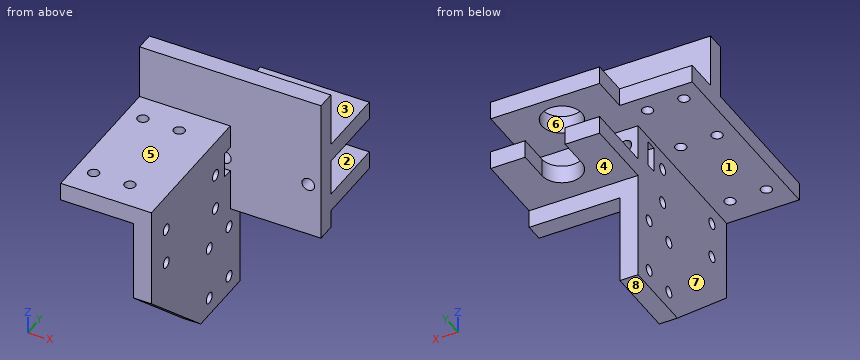
```python
from build123d import *

# Parameters (mm, degrees)
BOSS_EXTRUDE1_DEPTH = 10
SKETCH2_W           = 40
SKETCH2_H           = 10
BOSS_EXTRUDE2_DEPTH = 18.71
BOSS_EXTRUDE3_DEPTH = 80
SKETCH5_W           = 10
SKETCH5_H           = 90
BOSS_EXTRUDE4_DEPTH = 50
CUT_EXTRUDE1_DEPTH  = 10
SKETCH7_W           = 60
SKETCH7_H           = 10
BOSS_EXTRUDE5_DEPTH = 39
SKETCH8_R           = 3.5
CUT_EXTRUDE2_DEPTH  = 10
CUT_EXTRUDE3_DEPTH  = 10
SKETCH10_R          = 11
SKETCH10_R_2        = 3
CUT_EXTRUDE4_DEPTH  = 10
SKETCH11_R          = 3
CUT_EXTRUDE5_DEPTH  = 10
CUT_EXTRUDE6_START  = -10
CUT_EXTRUDE6_DEPTH  = 10


with BuildPart() as part:
    # Sketch1 → Boss-Extrude1 (new body)
    with BuildSketch(Plane(origin=(0, 0, 0), x_dir=(1, 0, 0), z_dir=(0, 1, 0))):
        Polygon((0, 0), (100, 0), (100, 80), (40, 80), (40, 40), (0, 40), align=None)
    extrude(amount=BOSS_EXTRUDE1_DEPTH)

    # Sketch2 → Boss-Extrude2 (add)
    with BuildSketch(Plane(origin=(0, 10, 0), x_dir=(1, 0, 0), z_dir=(0, 1, 0))):
        with Locations((20, 35)):
            Rectangle(SKETCH2_W, SKETCH2_H)
    extrude(amount=BOSS_EXTRUDE2_DEPTH)

    # Sketch3 → Boss-Extrude3 (add)
    with BuildSketch(Plane.XZ):
        Polygon((0, -30), (50, -30), (50, -80), (40, -80), (40, -40), (0, -40), align=None)
    extrude(amount=BOSS_EXTRUDE3_DEPTH)

    # Sketch5 → Boss-Extrude4 (add)
    with BuildSketch(Plane(origin=(0, 0, -80), x_dir=(-1, 0, 0), z_dir=(0, 0, -1))):
        with Locations((-45, -35)):
            Rectangle(SKETCH5_W, SKETCH5_H)
    extrude(amount=BOSS_EXTRUDE4_DEPTH)

    # Sketch6 → Cut-Extrude1 (cut)
    with BuildSketch(Plane.ZY.offset(-40)):
        Polygon((-85, -80), (-130, -30), (-130, -80), align=None)
    extrude(amount=-CUT_EXTRUDE1_DEPTH, mode=Mode.SUBTRACT)

    # Sketch7 → Boss-Extrude5 (add)
    with BuildSketch(Plane(origin=(0, 10, 0), x_dir=(1, 0, 0), z_dir=(0, 1, 0))):
        with Locations((70, 65)):
            Rectangle(SKETCH7_W, SKETCH7_H)
        with Locations((70, 35)):
            Rectangle(SKETCH7_W, SKETCH7_H)
    extrude(amount=BOSS_EXTRUDE5_DEPTH)

    # Sketch8 → Cut-Extrude2 (cut)
    with BuildSketch(Plane(origin=(0, 10, 0), x_dir=(1, 0, 0), z_dir=(0, 1, 0))):
        with Locations(Location((47, 50, 0), (0, 0, 270))):
            Circle(SKETCH8_R)
        with Locations(Location((93, 50, 0), (0, 0, 270))):
            Circle(SKETCH8_R)
    extrude(amount=-CUT_EXTRUDE2_DEPTH, mode=Mode.SUBTRACT)

    # Sketch9 → Cut-Extrude3 (cut)
    with BuildSketch(Plane(origin=(50, 0, 0), x_dir=(0, 0, -1), z_dir=(1, 0, 0))):
        Polygon((50, 0), (57, 0), (57, -6), (43, -6), (43, 0), align=None)
    extrude(amount=-CUT_EXTRUDE3_DEPTH, mode=Mode.SUBTRACT)

    # Sketch10 → Cut-Extrude4 (cut)
    with BuildSketch(Plane.XY.offset(-30)):
        with Locations((70, 32)):
            Circle(SKETCH10_R)
        with Locations((30, 18.71)):
            Circle(SKETCH10_R_2)
        with Locations((10, 18.71)):
            Circle(SKETCH10_R_2)
        with Locations((30, -15)):
            Circle(SKETCH10_R_2)
        with Locations((10, -15)):
            Circle(SKETCH10_R_2)
        with Locations((30, -65)):
            Circle(SKETCH10_R_2)
        with Locations((10, -65)):
            Circle(SKETCH10_R_2)
    extrude(amount=-CUT_EXTRUDE4_DEPTH, mode=Mode.SUBTRACT)

    # Sketch11 → Cut-Extrude5 (cut)
    with BuildSketch(Plane(origin=(50, 0, 0), x_dir=(0, 0, -1), z_dir=(1, 0, 0))):
        with Locations((50, -15)):
            Circle(SKETCH11_R)
        with Locations((70, -15)):
            Circle(SKETCH11_R)
        with Locations((70, -65)):
            Circle(SKETCH11_R)
        with Locations((50, -65)):
            Circle(SKETCH11_R)
        with Locations((90, -1.3)):
            Circle(SKETCH11_R)
        with Locations((120, -1.3)):
            Circle(SKETCH11_R)
        with Locations((90, -21.3)):
            Circle(SKETCH11_R)
        with Locations((120, -21.3)):
            Circle(SKETCH11_R)
    extrude(amount=-CUT_EXTRUDE5_DEPTH, mode=Mode.SUBTRACT)

    # Sketch12 → Cut-Extrude6 (cut)
    with BuildSketch(Plane(origin=(0, 0, -70), x_dir=(-1, 0, 0), z_dir=(0, 0, -1)).offset(CUT_EXTRUDE6_START)):
        with BuildLine():
            Line((-70, 49), (-59, 49))
            Line((-59, 49), (-59, 32))
            ThreePointArc((-59, 32), (-70, 21), (-81, 32))
            Line((-81, 32), (-81, 49))
            Line((-81, 49), (-70, 49))
        make_face()
    extrude(amount=CUT_EXTRUDE6_DEPTH, mode=Mode.SUBTRACT)


solid = part.part
```
The listing builds one solid part. Answer for the finished solid, in the listing's coordinates (mm). Face numbers are marked on the shaded views. A direction names the side the tool comes from. Coordinates: 2 decimals unless noted, no trailing zeros. Loops run counter-clockwise (first coordinate to the right, second up) from the corner with the lowest first, then second, coordinate; pieces in that order, holes last. Notation, with made-up numbers: (17, -7.75) -> (62, -7.75) arc R29 ccw to (62, 25.25) -> close; hole circle Ø4 at (-38, 87.25). An arc over 180 degrees is marked (long way). Use one line per item in the form item = value. Start each with the question number.
Item 1: The part is cut by section D-D on x = 84. Determine the outline of the cut face in (y, z).
Item 2: The part is cut by section B-B on y = -65. Determine the outline of the cut face in (x, z).
Item 3: Consider L1, parallel to Z at x = 46, y = -1; L2, parallel to Y at x = 46.25, z = -120; L3, parallel to Y at x = 30, z = -38. Determine where each line is inside the solid, lowest interval first. Write a range as [from, to].
Item 4: The mould has two halves that part along X. Classify the marked faces 6, 7 and 8: released by +X, released by -X, zero draft, split by the parting line, or undercut.
Item 5: A tool of negligible diameter and unlimited length cuts with its end or side. For the marked faces 1, 2, 3, 4 and 5, from which of +Z, -Z, +X, -X, +Y, -Y can it reach the whole face along a straight path? Write none if from no direction.
Item 6: The part is cut by section C-C on x = 62.5. Determine the outline of the cut face in (y, z).
Item 7: Flat-ended cylindrical pins translate along their axes: pin 1 Ø8 at (x, z) = (53.5, -45.5) entering from -Y; pin 2 Ø5 at (x, y) = (30, -15) entering from +Z; pin 3 Ø1.5 at (x, y) = (49, -63.5) entering from +Z; pin 4 Ø9.5 at (x, y) = (30, -65) entering from -Z. Find the tip coordinate at first contact, or state that the pin passes through.
Item 8: The part is cut by section A-A on y = -21.3. Determine the outline of the cut face in (x, z), then the cut area to 3 significant figures.
Answer key:
q1.outline = (0, -80) -> (10, -80) -> (10, -70) -> (49, -70) -> (49, -60) -> (10, -60) -> (10, -40) -> (49, -40) -> (49, -30) -> (10, -30) -> (10, 0) -> (0, 0) -> close
q2.outline = (0, -40) -> (7, -40) -> (7, -30) -> (0, -30) -> close; (13, -40) -> (27, -40) -> (27, -30) -> (13, -30) -> close; (33, -40) -> (40, -40) -> (40, -47) -> (50, -47) -> (50, -30) -> (33, -30) -> close; (40, -98.5) -> (50, -98.5) -> (50, -73) -> (40, -73) -> close; (40, -67) -> (50, -67) -> (50, -53) -> (40, -53) -> close
q3.L1 = [-130, -122.98], [-117.02, -92.98], [-87.02, -57], [-43, -30]
q3.L2 = [-41.11, -24.3], [-18.3, -4.3], [1.7, 10]
q3.L3 = [-80, -68], [-62, -18], [-12, 15.71], [21.71, 28.71]
q4.face_6 = undercut
q4.face_7 = released by -X
q4.face_8 = zero draft
q5.face_1 = -X, +Y
q5.face_2 = +X, -X, +Y
q5.face_3 = +Z, +X, -X, +Y
q5.face_4 = -Z, +X, -X, +Y
q5.face_5 = +Z, +X, -X, -Y
q6.outline = (0, -80) -> (10, -80) -> (10, -70) -> (23.95, -70) -> (23.95, -60) -> (10, -60) -> (10, -40) -> (23.95, -40) -> (23.95, -30) -> (10, -30) -> (10, 0) -> (0, 0) -> close; (40.05, -40) -> (49, -40) -> (49, -30) -> (40.05, -30) -> close
q7.pin_1 = -80
q7.pin_2 = through
q7.pin_3 = -30
q7.pin_4 = -40
q8.outline = (0, -40) -> (40, -40) -> (40, -87) -> (50, -87) -> (50, -30) -> (0, -30) -> close; (40, -130) -> (50, -130) -> (50, -123) -> (40, -123) -> close; (40, -117) -> (50, -117) -> (50, -93) -> (40, -93) -> close
q8.area = 1,280 mm2
